from build123d import *

# Parameters (mm, degrees)
F4_DEPTH = 22
F5_R     = 3
F6_DEPTH = 35.001


with BuildPart() as f1:
    # F0 (on Top) → F1 (revolve)
    with BuildSketch(Plane.XY):
        with BuildLine():
            ThreePointArc((0, -15), (15, 0), (0, 15))
            Line((0, 15), (0, -15))
        make_face()
    revolve(axis=Axis((0, 0, 0), (0, -1, 0)))

    # F3 (on offset) → F4 (cut)
    with BuildSketch(Plane.XY.offset(20)):
        Polygon((2.52286, -5.321201), (5.869725, -0.475739), (3.346865, 4.845461), (-2.52286, 5.321201), (-5.869725, 0.475739), (-3.346865, -4.845461), align=None)
    extrude(amount=-F4_DEPTH, mode=Mode.SUBTRACT)

    # F5 (on offset) → F6 (cut, through all)
    with BuildSketch(Plane.XY.offset(20)):
        Circle(F5_R)
    extrude(amount=-F6_DEPTH, mode=Mode.SUBTRACT)


solid = f1.part
Read the model definition and answer for the solid it produces. Units are mm, in the model's axes. A direction names the side the tool comes from. Give positions to 0.01 mm unless a question says otherwise; leave off trailing zeros. Loops run counter-clockwise (first coordinate to the right, second up) from the corner with the lowest first, then second, coordinate; pieces in that order, holes last. Notation, with made-up numbers: (81.25, 7.25) -> (96.25, 7.25) arc R14 ccw to (96.25, 18.25) -> close; hole circle Ø10 at (-13.5, -22). An arc over 180 degrees is marked (long way). Use a Markdown table: item, result.
Q1. Section D-D, the plane y = -10.25 is taken. Determine the outline of the cut face in (x, z), then the cut area to 3 significant figures.
Solved:
| item | result |
|---|---|
| outline | circle Ø21.9 at (0, 0) |
| area | 377 mm^2 |
Q2. A tool of negligible diameter and unlimited length cuts with its end or side. For faces 1 (the face through (-3, 0, -8)), 2 (the face through (-4.173, 2.932, 6.166)), from which of +Z, -Z, +X, -X, +Y, -Y can it reach the whole face along a straight path? Write none if from no direction.
Solved:
| item | result |
|---|---|
| face 1 | +Z, -Z |
| face 2 | +Z |
Q3. Find the intervals of material crossed by line 1 along Y through (x, z) = (-2.25, 9.75); line 2 along X through (y, z) = (0, -5.25); line 3 along Y through (x, z) = (1.5, -8.25), in increasing order.
Solved:
| item | result |
|---|---|
| line 1 | y = -11.17 to -4.93, 5.3 to 11.17 |
| line 2 | x = -14.05 to -3, 3 to 14.05 |
| line 3 | y = -12.44 to -2.6, 2.6 to 12.44 |
Q4. Section C-C, the plane y = 0 is taken. Determine the outline of the cut face in (x, z).
Solved:
| item | result |
|---|---|
| outline | (-5.64, -2) -> (-5.64, 13.9) arc R15 ccw to (-3, -14.7) -> (-3, -2) -> close; (3, -14.7) arc R15 ccw to (5.64, 13.9) -> (5.64, -2) -> (3, -2) -> close |
Q5. Each of these flat-tipped pins is pushed along its axis until it touches: pin 1 (8 mm diameter, centred on x = -2.5, z = 4.5, fed in from +Y); pin 2 (4 mm diameter, centred on x = -11.5, z = 3, fed in from -Y); pin 3 (4 mm diameter, centred on x = 0, y = -7.5, fed in from -Z). Where does it stop, or does it pass through?
Solved:
| item | result |
|---|---|
| pin 1 | stops at y = 14.96 |
| pin 2 | stops at y = -11.28 |
| pin 3 | stops at z = -13.96 |
Q6. Section B-B, the plane x = 0 is taken. Determine the outline of the cut face in (y, z), then the cut area to 3 significant figures.
Solved:
| item | result |
|---|---|
| outline | (-5.12, -2) -> (-5.12, 14.1) arc R15 ccw to (-3, -14.7) -> (-3, -2) -> close; (3, -14.7) arc R15 ccw to (5.12, 14.1) -> (5.12, -2) -> (3, -2) -> close |
| area | 459 mm^2 |
Q7. Section A-A, the plane z = 10.5 is taken. Determine the outline of the cut face in (x, y).
Solved:
| item | result |
|---|---|
| outline | circle Ø21.42 at (0, 0); hole (-5.87, 0.48) -> (-3.35, -4.85) -> (2.52, -5.32) -> (5.87, -0.48) -> (3.35, 4.85) -> (-2.52, 5.32) -> close |
